```python
from build123d import *

# Parameters (mm, degrees)
SKETCH1_W           = 26.9875
SKETCH1_H           = 26.9875
BOSS_EXTRUDE1_DEPTH = 19.05
SKETCH2_R           = 6.985
CUT_EXTRUDE1_DEPTH  = 20.05
CUT_EXTRUDE4_DEPTH  = 12.7
SKETCH4_R           = 2.3495
BOSS_EXTRUDE2_DEPTH = 3.175
CUT_EXTRUDE5_DEPTH  = 27.9875


with BuildPart() as part:
    # Sketch1 → Boss-Extrude1 (new body)
    with BuildSketch(Plane(origin=(0, 0, 0), x_dir=(1, 0, 0), z_dir=(0, 1, 0))):
        with Locations((13.49375, 13.49375)):
            Rectangle(SKETCH1_W, SKETCH1_H)
    extrude(amount=BOSS_EXTRUDE1_DEPTH)

    # Sketch2 → Cut-Extrude1 (cut, through all)
    with BuildSketch(Plane(origin=(0, 19.05, 0), x_dir=(1, 0, 0), z_dir=(0, 1, 0))):
        with Locations((13.49375, 13.49375)):
            Circle(SKETCH2_R)
    extrude(amount=-CUT_EXTRUDE1_DEPTH, mode=Mode.SUBTRACT)

    # Sketch3 → Cut-Extrude4 (cut)
    with BuildSketch(Plane(origin=(0, 19.05, 0), x_dir=(1, 0, 0), z_dir=(0, 1, 0))):
        Polygon((18.993011314, 23.01875), (7.994488686, 23.01875), (2.495227372, 13.49375), (7.994488686, 3.96875), (18.993011314, 3.96875), (24.492272628, 13.49375), align=None)
    extrude(amount=-CUT_EXTRUDE4_DEPTH, mode=Mode.SUBTRACT)

    # Sketch4 → Boss-Extrude2 (add)
    with BuildSketch(Plane(origin=(0, 0, -26.9875), x_dir=(-1, 0, 0), z_dir=(0, 0, -1))):
        with BuildLine():
            Line((0, 19.05), (-26.9875, 19.05))
            Line((-26.9875, 19.05), (-26.9875, 62.0875))
            ThreePointArc((-26.9875, 62.0875), (-13.49375, 75.58125), (0, 62.0875))
            Line((0, 62.0875), (0, 19.05))
        make_face()
        with Locations((-13.49375, 62.0875)):
            Circle(SKETCH4_R, mode=Mode.SUBTRACT)
    boss_extrude2 = extrude(amount=-BOSS_EXTRUDE2_DEPTH)

    # Mirror1: Boss-Extrude2 across plane
    add(boss_extrude2.mirror(Plane(origin=(0, 0, -13.49375), x_dir=(1, 0, 0), z_dir=(0, 0, -1))))

    # Sketch6 → Cut-Extrude5 (cut, through all)
    with BuildSketch(Plane(origin=(0, 0, -26.9875), x_dir=(-1, 0, 0), z_dir=(0, 0, -1))):
        Polygon((-20.6375, 46.83125), (-13.49375, 53.975), (-6.35, 46.83125), (-6.35, 19.05), (-20.6375, 19.05), align=None)
    extrude(amount=-CUT_EXTRUDE5_DEPTH, mode=Mode.SUBTRACT)


solid = part.part
```
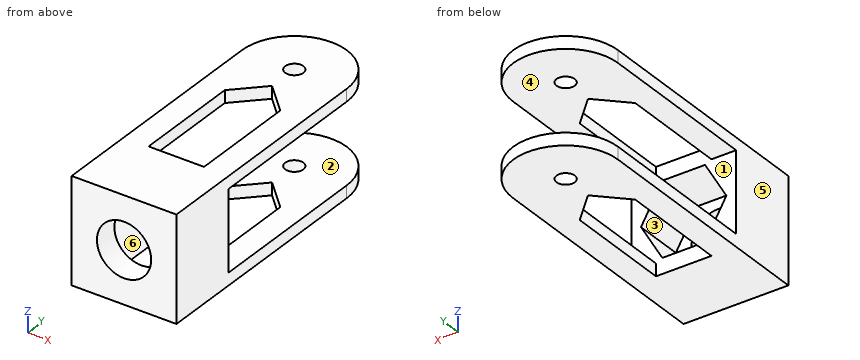
Geometry: final body of the model. Coordinates: model frame, mm. Face numbers are marked on the shaded views. A direction names the side the tool comes from. Coordinates: 2 decimals unless noted, no trailing zeros. Order: outer loops, then holes, each group sorted by start corner. A loop starts at its lowest first (then second) coordinate and runs counter-clockwise, first axis right, second up. Notation, with made-up numbers: M 24,-23 L 29,-23 A22 cw 29,16 Z; hole C 80,75 d7. An arc over 180 degrees is marked long. Answer in a Markdown table with one row per item. Add a question column.
Q1. Section query D-D on z = -10.75. Return the cut outline in (x, y).
Q2. Section query A-A on y = 11. Return the cut outline in (x, z).
Q3. Reachability of the marked faces 1, 2 and 3 from +Z, -Z, +X, -X, +Y, -Y: full face, straight path, thin tool, end or side. Return the list, or none.
Q4. Line query: L1, parallel to Z at x = 25, y = 47 (1 decimal); L2, parallel to X at y = 10.5, z = -5.5; L3, parallel to X at y = 14.5, z = -6.25. Output: solid intervals per line, ascending.
Q5. Contact query for flat-ended pins moving along their axis: P1, Ø15, axis at x = 19, z = -14, coming from the +Y side; P2, Ø1, axis at x = 16.5, z = -7, coming from the +Y side; P3, Ø13.5, axis at x = 19, z = -8.5, coming from the +Y side; P4, Ø4, axis at x = 13.49, y = 62.09, coming from the -Z side. Output: stop coordinate, or through.
Q6. Mould query, pull axis X, two halves, no side actions, for the marked faces 4, 5 and 6. Classes: released by +X, released by -X, zero draft, split by the parting line, or undercut.
Q7. Section query B-B on x = 12.5. Count the separate pieces of the cut face and the enclosed holes in it, and give its area (3 significant figures).
Completed:
| question | item | result |
|---|---|---|
| 1 | outline | M 0,0 L 7.07,0 L 7.07,6.35 L 4.08,6.35 L 4.08,19.05 L 0,19.05 Z; M 19.92,0 L 26.99,0 L 26.99,19.05 L 22.91,19.05 L 22.91,6.35 L 19.92,6.35 Z |
| 2 | outline | M 0,-26.99 L 26.99,-26.99 L 26.99,0 L 0,0 Z; hole M 2.5,-13.49 L 7.99,-23.02 L 18.99,-23.02 L 24.49,-13.49 L 18.99,-3.97 L 7.99,-3.97 Z |
| 3 | face 1 | none |
| 3 | face 2 | +X, -X, +Y |
| 3 | face 3 | +Y |
| 4 | L1 | z = -27 to -23.8, -3.2 to 0 |
| 4 | L2 | x = 0 to 7.11, 19.88 to 26.99 |
| 4 | L3 | x = 0 to 6.68, 20.31 to 26.99 |
| 5 | P1 | stops at y = 19.05 |
| 5 | P2 | stops at y = 6.35 |
| 5 | P3 | stops at y = 75.51 |
| 5 | P4 | passes through |
| 6 | face 4 | zero draft |
| 6 | face 5 | released by -X |
| 6 | face 6 | undercut |
| 7 | separate pieces | 6 |
| 7 | enclosed holes | 0 |
| 7 | area | 301 mm2 |
